Autodesk Inventor part; units mm, degrees
ref_plane "YZ Plane" through (0, 0, 0) normal (1, 0, 0) x (0, 1, 0)
ref_plane "XZ Plane" through (0, 0, 0) normal (0, 1, 0) x (-1, 0, 0)
ref_plane "XY Plane" through (0, 0, 0) normal (0, 0, 1) x (1, 0, 0)
sketch "Sketch1" plane through (0, 0, 0) normal (0, 1, 0) x (-1, 0, 0)
  circle A0 centre (0, 0) radius 30
  dimension "d0" = 60
extrude "Extrusion1" add sketch "Sketch1" against normal blind 6
sketch "Sketch2" plane through (0, 0, 0) normal (0, 1, 0) x (1, 0, 0)
  line L0 (-10, -18) -> (10, -18)
  line L1 (10, -32) -> (-10, -32)
  line L2 (-10, -18) -> (10, -32) construction
  line L3 (10, -18) -> (-10, -32) construction
  arc A0 (-7.5, -25) -> (-12.5, -25) centre (-10, -25) ccw
  arc A1 (12.5, -25) -> (7.5, -25) centre (10, -25) ccw
  line L4 (-12.5, -25) -> (12.5, -25)
  line L5 (-10, -32) -> (-10, -27.5)
  line L6 (-10, -25) -> (-10, -18)
  line L7 (10, -18) -> (10, -25)
  line L8 (10, -27.5) -> (10, -32)
  point P0 (0, 0)
  point P1 (0, -25)
  dimension "d3" = 20
  dimension "d4" = 25
  dimension "d5" = 14
  dimension "d6" = 5
  dimension "d7" = 5
revolve "Revolution1" cut sketch "Sketch2" angle 360 about axis through (-12.5, 0, 25) along (1, 0, 0)
sketch "Sketch3" plane through (0, -6, 0) normal (0, -1, 0) x (1, 0, 0)
  arc A0 (9.04, 28.6056) -> (-9.04, 28.6056) centre (0, 0) ccw
  line L0 (-9.04, 28.6056) -> (9.04, 28.6056)
  arc A1 (9.04, 28.6056) -> (-9.04, 28.6056) centre (0, 0) ccw
extrude "Extrusion2" cut sketch "Sketch3" against normal through all
fillet "Fillet1" radius 6 1 edges at (0, -6, -30)
pattern_circular "Circular Pattern1" count 4 over 360 about axis through (0, -10, 0) along (0, 1, 0) of "Revolution1"
properties part number "wheel_cover"
Geometry check sheet. Reference: the model listing, model coordinates, mm. A direction names the side the tool comes from. Coordinates: 2 decimals unless noted, no trailing zeros. Order: outer loops, then holes, each group sorted by start corner. A loop starts at its lowest first (then second) coordinate and runs counter-clockwise, first axis right, second up. Notation, with made-up numbers: (72.25, 70.25) - (88.25, 70.25) arc R24 ccw to (88.25, 101.25) - close; hole circle Ø5 at (77.25, 64.25). An arc over 180 degrees is marked (long way). Use one line per item in the form item = value.
1. Gauge pin test, flat ends, axial feed: pin 1 (3 mm diameter, centred on y = -2.5, z = 23, fed in from -X); pin 2 (3 mm diameter, centred on x = -22, y = -3, fed in from +Z); pin 3 (2 mm diameter, centred on x = 16, y = -5.5, fed in from -Z). Record the tip position at first contact, or that the pin passes through.
Here are the results:
pin_1 = -20.35
pin_2 = 21.1
pin_3 = -23.1
2. Access from +Z, -Z, +X, -X, +Y, -Y to the whole of each face (thin tool, end or side, straight path). Record for faces 1 (the face through (22, -3, 10)), 2 (the face through (-22, -3, 10)), 3 (the face through (10, -3, -22)).
Here are the results:
face_1 = +X, +Y
face_2 = -X, +Y
face_3 = -Z, +Y
3. Section check D-D (y = -5.25). Record the boundary of the cut face in (x, z), then the cut area to 3 significant figures.
Here are the results:
outline = (-24.98, -10) arc R26.9 ccw to (-10, -24.98) - (-10, -20.37) - (10, -20.37) - (10, -24.98) arc R26.9 ccw to (24.98, -10) - (20.37, -10) - (20.37, 10) - (24.98, 10) arc R26.9 ccw to (10, 24.98) - (10, 20.37) - (-10, 20.37) - (-10, 24.98) arc R26.9 ccw to (-24.98, 10) - (-20.37, 10) - (-20.37, -10) - close
area = 1,800 mm²
4. Draft check along Z on faces 4 (the face through (-18.93, -3.49, 0.14)), 5 (the face through (0.14, -3.49, 18.93)), 6 (the face through (10, -3, 22)). Enter one of: pulls with the +Z half, pulls with the -Z half, needs draft (parallel to the pull), parting line crosses it, or undercut.
Here are the results:
face_4 = undercut
face_5 = pulls with the +Z half
face_6 = needs draft
5. Scan lines: line 1 (Z direction, x = -11, y = -1.25); line 2 (X direction, y = -0.5, z = -20.5); line 3 (Z direction, x = 24.5, y = -4). Record each from-to range of solid material in increasing order.
Here are the results:
line_1 = -27.77 to -26.92, -23.08 to 23.08, 26.92 to 27.77
line_2 = -21.87 to -10, 10 to 21.87
line_3 = -14.51 to -10, 10 to 14.51
6. Section check C-C (x = 3.5). Record the boundary of the cut face in (y, z).
Here are the results:
outline = (-6, -21.39) arc R7 cw to (0, -18) - (0, 18) arc R7 cw to (-6, 21.39) - close
7. Section check B-B (z = 5). Record the boundary of the cut face in (x, y).
Here are the results:
outline = (-21.39, -6) - (21.39, -6) arc R7 cw to (18, 0) - (-18, 0) arc R7 cw to start
